Source: CAD feature listing. Evaluate the final solid. Frame: model axes, mm. A direction names the side the tool comes from. Coordinates: 2 decimals unless noted, no trailing zeros. Write each loop counter-clockwise with the first axis right and the second up, starting at its lowest first coordinate (ties: lowest second). Pieces come first, ordered by that corner, then holes. Notation, with made-up numbers: M 86.25,0.25 L 136.25,0.25 A30 cw 136.25,38.25 Z; hole C 20,22.5 d4. An arc over 180 degrees is marked long. Answer as CSV lines item,"result". Start each with the question number.
1. Line query: probe 1 along Y at (x, z) = (0, 8); probe 2 along Y at (x, z) = (15.5, 3). Output: solid intervals per line, ascending. Write a range as [from, to].
2. Reachability of faces 1 (the face through (0, 1, 2)), 2 (the face through (25, 2, 0)) from +Z, -Z, +X, -X, +Y, -Y: full face, straight path, thin tool, end or side. Return the list, or none.
3. Contact query for flat-ended pins moving along their axis: pin 1 Ø6 at (x, z) = (-18.5, 5.5) entering from +Y; pin 2 Ø0.7 at (x, z) = (-9.5, 8) entering from +Y; pin 3 Ø2 at (x, z) = (5, -2) entering from +Y. Output: stop coordinate, or through.
4. Section B-B on z = 1. Return the cut outline in (x, y), plus the area to 3 significant figures.
5. Mould query, pull axis Z, two halves, no side actions, for faces 3 (the face through (0, 3, 10)), 4 (the face through (0, 1, -2)), 5 (the face through (-25, 2, 0)). Classes: pulls with the +Z half, pulls with the -Z half, needs draft (parallel to the pull), parting line crosses it, or undercut.
6. Section A-A on y = 2.45. Return the cut outline in (x, z) (3 decimals), plus the area to 3 significant figures.
```python
from build123d import *

# Parameters (mm, degrees)
SKETCH_1_W          = 50
SKETCH_1_H          = 20
EXTRUDE_1_DEPTH     = 6
SKETCH_2_W          = 50
SKETCH_2_H          = 2.34
CUT_EXTRUDE_1_DEPTH = 5
FILLET_1_R          = 0.5


with BuildPart() as part:
    # 草图1 → 凸台-拉伸1 (new body)
    with BuildSketch(Plane(origin=(0, 0, 0), x_dir=(1, 0, 0), z_dir=(0, 1, 0))):
        Rectangle(SKETCH_1_W, SKETCH_1_H)
    extrude(amount=EXTRUDE_1_DEPTH)

    # 草图2 → 切除-拉伸1 (cut)
    with BuildSketch(Plane(origin=(0, 6, 0), x_dir=(1, 0, 0), z_dir=(0, 1, 0))):
        with Locations((0, 1.595)):
            Rectangle(SKETCH_2_W, SKETCH_2_H)
        with Locations((0, -1.595)):
            Rectangle(SKETCH_2_W, SKETCH_2_H)
        with Locations((0, 4.785)):
            Rectangle(SKETCH_2_W, SKETCH_2_H)
        with Locations((0, -4.785)):
            Rectangle(SKETCH_2_W, SKETCH_2_H)
        with Locations((0, 7.975)):
            Rectangle(SKETCH_2_W, SKETCH_2_H)
        with Locations((0, -7.975)):
            Rectangle(SKETCH_2_W, SKETCH_2_H)
    extrude(amount=-CUT_EXTRUDE_1_DEPTH, mode=Mode.SUBTRACT)

    # 圆角1
    # the kernel refuses this fillet: 0.5 mm, written as the material it takes off along each edge
    with BuildSketch(Plane(origin=(26.25, 6, 10), x_dir=(0, 0, -1), z_dir=(-1, 0, 0)), Plane(origin=(26.25, 6, 6.805), x_dir=(0, 0, -1), z_dir=(-1, 0, 0)), Plane(origin=(26.25, 6, 3.615), x_dir=(0, 0, -1), z_dir=(-1, 0, 0)), Plane(origin=(26.25, 6, 0.425), x_dir=(0, 0, -1), z_dir=(-1, 0, 0)), Plane(origin=(26.25, 6, -2.765), x_dir=(0, 0, -1), z_dir=(-1, 0, 0)), Plane(origin=(26.25, 6, -5.955), x_dir=(0, 0, -1), z_dir=(-1, 0, 0)), Plane(origin=(26.25, 6, -9.145), x_dir=(0, 0, -1), z_dir=(-1, 0, 0))) as fillet_1_piece_1:
        with BuildLine():
            CenterArc((FILLET_1_R, FILLET_1_R), FILLET_1_R, 180, 90)
            Line((0, FILLET_1_R), (0, 0))
            Line((0, 0), (FILLET_1_R, 0))
        make_face()
    extrude(amount=52.5, mode=Mode.SUBTRACT)
    with BuildSketch(Plane(origin=(-26.25, 6, -10), x_dir=(0, -1, 0), z_dir=(1, 0, 0)), Plane(origin=(-26.25, 6, 9.145), x_dir=(0, -1, 0), z_dir=(1, 0, 0)), Plane(origin=(-26.25, 6, 5.955), x_dir=(0, -1, 0), z_dir=(1, 0, 0)), Plane(origin=(-26.25, 6, 2.765), x_dir=(0, -1, 0), z_dir=(1, 0, 0)), Plane(origin=(-26.25, 6, -0.425), x_dir=(0, -1, 0), z_dir=(1, 0, 0)), Plane(origin=(-26.25, 6, -3.615), x_dir=(0, -1, 0), z_dir=(1, 0, 0)), Plane(origin=(-26.25, 6, -6.805), x_dir=(0, -1, 0), z_dir=(1, 0, 0))) as fillet_1_piece_2:
        with BuildLine():
            CenterArc((FILLET_1_R, -FILLET_1_R), FILLET_1_R, 90, 90)
            Line((0, -FILLET_1_R), (0, 0))
            Line((0, 0), (FILLET_1_R, 0))
        make_face()
    extrude(amount=52.5, mode=Mode.SUBTRACT)


solid = part.part
```
Values:
1,probe 1,"[0, 1]"
1,probe 2,"[0, 5.92]"
2,face 1,"+X, -X, +Y"
2,face 2,"+Z, -Z, +X, +Y, -Y"
3,pin 1,"y = 5.99"
3,pin 2,"y = 1"
3,pin 3,"y = 5.92"
4,outline,"M -25,0 L 25,0 L 25,1 L -25,1 Z"
4,area,"50.0 mm²"
5,face 3,"pulls with the +Z half"
5,face 4,"undercut"
5,face 5,"needs draft"
6,outline,"M -25,-10 L 25,-10 L 25,-9.145 L -25,-9.145 Z; M -25,-6.805 L 25,-6.805 L 25,-5.955 L -25,-5.955 Z; M -25,-3.615 L 25,-3.615 L 25,-2.765 L -25,-2.765 Z; M -25,-0.425 L 25,-0.425 L 25,0.425 L -25,0.425 Z; M -25,2.765 L 25,2.765 L 25,3.615 L -25,3.615 Z; M -25,5.955 L 25,5.955 L 25,6.805 L -25,6.805 Z; M -25,9.145 L 25,9.145 L 25,10 L -25,10 Z"
6,area,"298 mm²"
